Read the model definition and answer for the solid it produces. Units are mm, in the model's axes. Give positions to 0.01 mm unless a question says otherwise; leave off trailing zeros. Order: outer loops, then holes, each group sorted by start corner. A loop starts at its lowest first (then second) coordinate and runs counter-clockwise, first axis right, second up.
```python
from build123d import *

# Parameters (mm, degrees)
SKETCH_1_W          = 78
SKETCH_1_H          = 100
EXTRUDE_1_DEPTH     = 3
SKETCH_3_R          = 2.75
CUT_EXTRUDE_1_DEPTH = 10


with BuildPart() as part:
    # 草图1 → 凸台-拉伸1 (new body)
    with BuildSketch(Plane.XY):
        with Locations((39, 50)):
            Rectangle(SKETCH_1_W, SKETCH_1_H)
    extrude(amount=EXTRUDE_1_DEPTH)

    # 草图3 → 切除-拉伸1 (cut)
    with BuildSketch(Plane.XY.offset(3)):
        with Locations((10, 95)):
            Circle(SKETCH_3_R)
        with Locations((10, 5)):
            Circle(SKETCH_3_R)
        with Locations((68, 5)):
            Circle(SKETCH_3_R)
        with Locations((68, 95)):
            Circle(SKETCH_3_R)
    extrude(amount=-CUT_EXTRUDE_1_DEPTH, mode=Mode.SUBTRACT)


solid = part.part
```
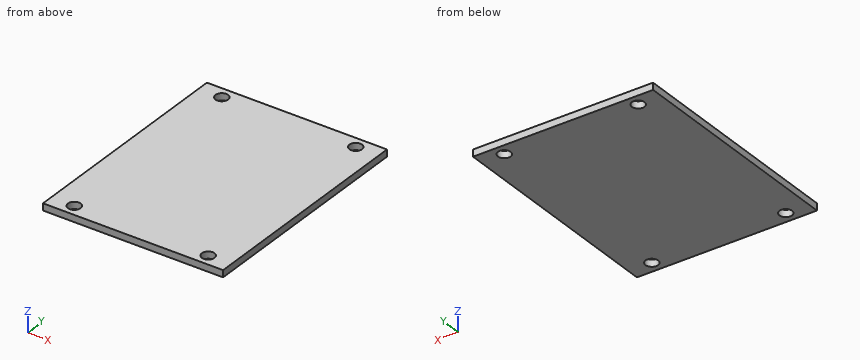
1) The part is cut by section A-A on y = 95. Determine the outline of the cut face in (x, z), and give its area (3 significant figures).
Final values:
outline: (0, 0) - (7.25, 0) - (7.25, 3) - (0, 3) - close; (12.75, 0) - (65.25, 0) - (65.25, 3) - (12.75, 3) - close; (70.75, 0) - (78, 0) - (78, 3) - (70.75, 3) - close
area: 201 mm2
2) Given pin 1 (4.5 mm diameter, centred on x = 68, y = 5, fed in from +Z), flat-ended and moving along its own axis, determine where the tip first touches the part or whether it passes through.
Final values:
pin 1: passes through
3) Consider L1, parallel to Y at x = 10, z = 1.4; L2, parallel to Y at x = 7.5, z = 1. Determine where each line is inside the solid, lowest interval first.
Final values:
L1: y = 0 to 2.25, 7.75 to 92.25, 97.75 to 100
L2: y = 0 to 3.85, 6.15 to 93.85, 96.15 to 100
4) The part is cut by section B-B on x = 68. Determine the outline of the cut face in (y, z), and give its area (3 significant figures).
Final values:
outline: (0, 0) - (2.25, 0) - (2.25, 3) - (0, 3) - close; (7.75, 0) - (92.25, 0) - (92.25, 3) - (7.75, 3) - close; (97.75, 0) - (100, 0) - (100, 3) - (97.75, 3) - close
area: 267 mm2
